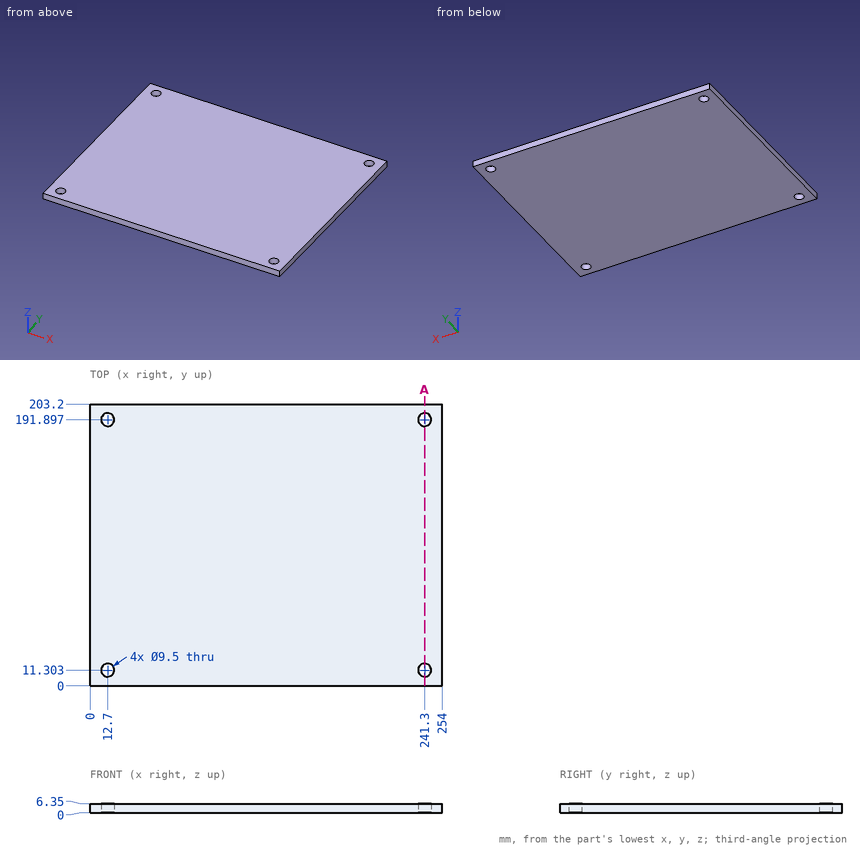
The drawing under review shows one solid part. Ordinate dimensions are in mm from its lowest x, y, z. Give positions to 0.01 mm unless a question says otherwise; leave off trailing zeros. Order: outer loops, then holes, each group sorted by start corner. A loop starts at its lowest first (then second) coordinate and runs counter-clockwise, first axis right, second up. Notation, with made-up numbers: (77.5, 17.5) - (111.5, 17.5) arc R21 cw to (111.5, 33.5) - close; hole circle Ø11 at (-3, 33.5). An arc over 180 degrees is marked (long way). Answer as a JSON object with one key per item and string values. Group by question number.
Item 1: Wall thickness on line 1 along Y through (x, z) = (241.3, 3); line 2 along X through (y, z) = (193.5, 1.75); line 3 along X through (y, z) = (194, 0.5): over which ranges is each line inside the solid? List them lowest first.
Item 2: Clearance check with a flat-ended pin moving along its axis: pin 1 Ø7.5 at (x, y) = (12.7, 11.303) entering from -Z. State where the tip first meets the part, or that it passes through.
Item 3: Take a section at A-A on x = 241.3. Give the boundary of the cut face in (y, z), and give its area (3 significant figures).
Reported:
{
 "1": {"line 1": "0 to 6.55, 16.05 to 187.15, 196.65 to 203.2", "line 2": "0 to 8.23, 17.17 to 236.83, 245.77 to 254", "line 3": "0 to 8.44, 16.96 to 237.04, 245.56 to 254"},
 "2": {"pin 1": "through"},
 "3": {"outline": "(0, 0) - (6.55, 0) - (6.55, 6.35) - (0, 6.35) - close; (16.05, 0) - (187.15, 0) - (187.15, 6.35) - (16.05, 6.35) - close; (196.65, 0) - (203.2, 0) - (203.2, 6.35) - (196.65, 6.35) - close", "area": "1,170 mm^2"}
}
